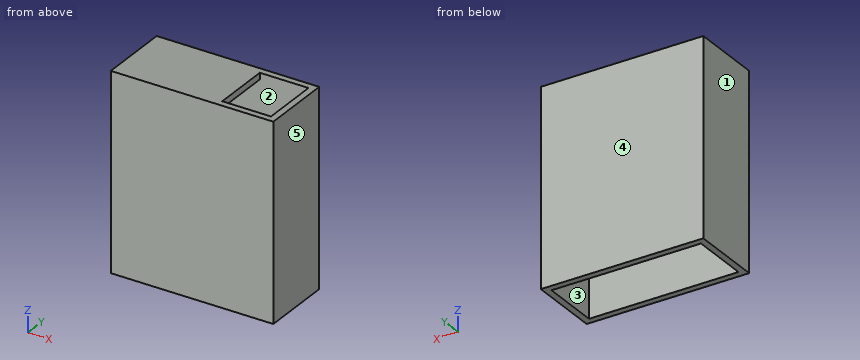
Autodesk Inventor part; units mm, degrees
ref_plane "YZ Plane" through (0, 0, 0) normal (1, 0, 0) x (0, 1, 0)
ref_plane "XZ Plane" through (0, 0, 0) normal (0, 1, 0) x (-1, 0, 0)
ref_plane "XY Plane" through (0, 0, 0) normal (0, 0, 1) x (1, 0, 0)
sketch "Skizze1" plane through (0, 0, 0) normal (0, 1, 0) x (-1, 0, 0)
  line L0 (0, 0) -> (-100, 0)
  line L1 (-100, 0) -> (-100, -120)
  line L2 (-100, -120) -> (0, -120)
  line L3 (0, -120) -> (0, 0)
  dimension "d0" = 100
  dimension "d1" = 120
extrude "Extrusion1" add sketch "Skizze1" along normal blind 4
sketch "Skizze2" plane through (0, 0, 0) normal (0, -1, 0) x (1, 0, 0)
  line L0 (100, 0) -> (100, -120)
  line L1 (100, -120) -> (0, -120)
  line L2 (0, -120) -> (0, 0)
  line L3 (0, 0) -> (100, 0)
  line L4 (4, -116) -> (96, -116)
  line L5 (96, -116) -> (96, -4)
  line L6 (96, -4) -> (4, -4)
  line L7 (4, -4) -> (4, -116)
  line L8 (4, -116) -> (4, -120)
  line L9 (96, -116) -> (96, -120)
  dimension "d4" = 4
extrude "Extrusion2" add sketch "Skizze2" against normal blind 40 contours L0 L1 L9 L5 L6 L7 L8 L2 L3
sketch "Skizze3" plane through (0, 40, 0) normal (0, 1, 0) x (1, 0, 0)
  line L0 (100, 120) -> (0, 120)
  line L1 (100, 0) -> (100, 120)
  line L2 (0, 0) -> (100, 0)
  line L3 (0, 120) -> (0, 0)
extrude "Extrusion3" add sketch "Skizze3" along normal blind 4
sketch "Skizze4" plane through (0, 0, 0) normal (0, 0, 1) x (1, 0, 0)
  line L0 (4, 4) -> (96, 4) construction
  line L1 (4, 4) -> (4, 40) construction
  line L2 (96, 40) -> (4, 40) construction
  line L3 (96, 4) -> (96, 40) construction
  line L4 (96, 40) -> (66, 40)
  line L5 (66, 40) -> (66, 4)
  line L6 (66, 4) -> (96, 4)
  line L7 (96, 4) -> (96, 40)
  point P0 (0, 0)
  dimension "d9" = 30
extrude "Extrusion4" cut sketch "Skizze4" against normal blind 4
properties part number "Schutzbox technik"
CAD build for the part. Positions are in the model's coordinates, mm. Face numbers are marked on the shaded views. A direction names the side the tool comes from. Coordinates: 2 decimals unless noted, no trailing zeros. Loops run counter-clockwise (first coordinate to the right, second up) from the corner with the lowest first, then second, coordinate; pieces in that order, holes last. Notation, with made-up numbers: (7.25, -9) -> (20.25, -9) arc R38 ccw to (20.25, 30) -> close; hole circle Ø5 at (21, -29.75). An arc over 180 degrees is marked (long way). One line per item, written item: value.
1. Which spindle directions (+Z, -Z, +X, -X, +Y, -Y) get a long thin tool onto all of the face, cutting with end or side? Do the marked faces 1 and 2. Say none if no direction does.
Answers:
face 1: +Z, -Z, -X, +Y, -Y
face 2: -Z
2. Drill centre lines: line 1 (Y direction, x = 14, z = -78.5); line 2 (X direction, y = 11.5, z = -24); line 3 (Z direction, x = 37.5, y = 14). Where is each one in solid material? Low to high. Write a range as [from, to].
Answers:
line 1: y = [0, 4], [40, 44]
line 2: x = [0, 4], [96, 100]
line 3: z = [-4, 0]
3. Slice it at D-D on x = 57.5. Write the cut outline in (y, z), and give its area (3 significant figures).
Answers:
outline: (0, -120) -> (4, -120) -> (4, -4) -> (40, -4) -> (40, -120) -> (44, -120) -> (44, 0) -> (0, 0) -> close
area: 1,100 mm^2
4. Slice it at C-C on y = 36. Write the cut outline in (x, z), and give its area (3 significant figures).
Answers:
outline: (0, -120) -> (4, -120) -> (4, -4) -> (66, -4) -> (66, 0) -> (0, 0) -> close; (96, -120) -> (100, -120) -> (100, 0) -> (96, 0) -> close
area: 1,210 mm^2
5. Pull direction X, two halves, no side cores. Call the marked faces 3, 4 and 5: pulls with the +X half, pulls with the -X half, needs draft (parallel to the pull), parting line crosses it, or undercut.
Answers:
face 3: undercut
face 4: needs draft
face 5: pulls with the +X half
6. Slice it at A-A on z = -61. Write the cut outline in (x, y).
Answers:
outline: (0, 0) -> (100, 0) -> (100, 44) -> (0, 44) -> close; hole (4, 4) -> (96, 4) -> (96, 40) -> (4, 40) -> close
7. Slice it at B-B on x = 88. Write the cut outline in (y, z).
Answers:
outline: (0, -120) -> (4, -120) -> (4, 0) -> (0, 0) -> close; (40, -120) -> (44, -120) -> (44, 0) -> (40, 0) -> close
